from build123d import *

# Parameters (mm, degrees)
F1_DEPTH = 60
F2_R     = 11.5
F3_DEPTH = 2.5
F5_T     = -2.5
F4_R     = 1
F6_DEPTH = 25
F7_SIZE  = 1.5
F8_R     = 3.5
F8_R_2   = 5
F8_R_3   = 10
F9_DEPTH = 3


with BuildPart() as f1:
    # F0 (on Right) → F1 (new body)
    with BuildSketch(Plane.YZ):
        Polygon((30, 63), (-30, 63), (-30, 3), (0, 3), (30, 3), align=None)
    extrude(amount=F1_DEPTH)

    # F2 (on face) → F3 (cut)
    with BuildSketch(Plane(origin=(0, 0, 0), x_dir=(0, -1, 0), z_dir=(-1, 0, 0))):
        with Locations((0, 40)):
            Circle(F2_R)
    extrude(amount=-F3_DEPTH, mode=Mode.SUBTRACT)

    # F5
    f5_openings = [f1.faces().sort_by_distance(p)[0] for p in [
        (60, 0, 33),
    ]]
    offset(amount=F5_T, openings=f5_openings, kind=Kind.INTERSECTION)

    # F4 (on face) → F6 (cut)
    with BuildSketch(Plane(origin=(0, 0, 0), x_dir=(0, -1, 0), z_dir=(-1, 0, 0))):
        with Locations((0, 49.5)):
            Circle(F4_R)
        with Locations((-8.227241336, 44.75)):
            Circle(F4_R)
        with Locations((-8.227241336, 35.25)):
            Circle(F4_R)
        with Locations((0, 30.5)):
            Circle(F4_R)
        with Locations((8.227241336, 35.25)):
            Circle(F4_R)
        with Locations((8.227241336, 44.75)):
            Circle(F4_R)
    extrude(amount=-F6_DEPTH, mode=Mode.SUBTRACT)

    # F7
    f7_edges = [f1.edges().sort_by_distance(p)[0] for p in [
        (30, -30, 63),
        (30, 30, 63),
        (30, 30, 3),
        (30, -30, 3),
        (0, -30, 33),
        (0, 0, 63),
        (0, 30, 33),
        (0, 0, 3),
    ]]
    chamfer(f7_edges, length=F7_SIZE)

    # F8 (on face) → F9 (cut)
    with BuildSketch(Plane(origin=(0, 30, 0), x_dir=(-1, 0, 0), z_dir=(0, 1, 0))):
        with Locations((-50.75, 22)):
            Circle(F8_R)
        with Locations((-50.75, 33)):
            Circle(F8_R_2)
        with Locations((-30.75, 33)):
            Circle(F8_R_3)
    extrude(amount=-F9_DEPTH, mode=Mode.SUBTRACT)


solid = f1.part
Build history of the part. All positions in model axes, mm. A direction names the side the tool comes from. Coordinates: 2 decimals unless noted, no trailing zeros. Order: outer loops, then holes, each group sorted by start corner. A loop starts at its lowest first (then second) coordinate and runs counter-clockwise, first axis right, second up. Notation, with made-up numbers: (8, 35.5) - (22, 35.5) arc R24 ccw to (22, 45.5) - close; hole circle Ø2 at (-35, 45.5). An arc over 180 degrees is marked (long way). Write each question's results on one line, items separated by ' | '. Start each with the question number.
Item 1: Band-saw the part on A-A on x = 50.75. Write the cut outline in (y, z).
Item 2: Band-saw the part on C-C on x = 30.75. Write the cut outline in (y, z).
Item 3: Band-saw the part on B-B on z = 44.75. Write the cut outline in (x, y), and give its area (3 significant figures).
Item 4: Flat gauge pins, fed straight in: pin 1 (14 mm diameter, centred on y = 5.5, z = 41.5, fed in from +X); pin 2 (8 mm diameter, centred on y = -0.5, z = 14, fed in from +X); pin 3 (18.5 mm diameter, centred on y = 0, z = 40.5, fed in from -X). Where does each tip first touch, or does it go through?
Item 5: Tool access for faces 4 (the face through (2.5, 0, 40)), 5 (the face through (0, 0, 27)), 6 (the face through (30, -30, 33)), 7 (the face through (55.745, 28.768, 33.22)), 8 (the face through (2.5, -6, 27)): list every direction of +Z, -Z, +X, -X, +Y, -Y with a clear straight run to the whole face (end or side of a thin tool).
Item 6: Mould opens along Z. For faces 1 (the face through (30, 0, 3)), 2 (the face through (60, -2, 4)), 3 (the face through (31, 0, 5.5)) say: released by +Z, released by -Z, zero draft, split by the parting line, or undercut.
Item 7: Wall check: probe 1 along Z at (x, y) = (3.25, 0); probe 2 along Z at (x, y) = (50.5, -1.5); probe 3 along Y at (x, z) = (8.5, 7.5). Give the ranges that are in metal, low to high. Write a range as [from, to].
Item 8: Band-saw the part on D-D on y = 25.5. Write the cut outline in (x, z), and give its area (3 significant figures).
Numbers:
1) outline: (-30, 4.5) - (-28.5, 3) - (28.5, 3) - (30, 4.5) - (30, 18.5) - (27.5, 18.5) - (27.5, 5.5) - (-27.5, 5.5) - (-27.5, 60.5) - (27.5, 60.5) - (27.5, 38) - (30, 38) - (30, 61.5) - (28.5, 63) - (-28.5, 63) - (-30, 61.5) - close; (27.5, 25.5) - (30, 25.5) - (30, 28) - (27.5, 28) - close
2) outline: (-30, 4.5) - (-28.5, 3) - (28.5, 3) - (30, 4.5) - (30, 23) - (27.5, 23) - (27.5, 5.5) - (-27.5, 5.5) - (-27.5, 60.5) - (27.5, 60.5) - (27.5, 43) - (30, 43) - (30, 61.5) - (28.5, 63) - (-28.5, 63) - (-30, 61.5) - close
3) outline: (0, -28.5) - (1.5, -30) - (60, -30) - (60, -27.5) - (2.5, -27.5) - (2.5, -13.17) - (5, -13.17) - (5, -9.23) - (2.5, -9.23) - (2.5, -10.47) - (0, -10.47) - close; (0, 10.47) - (2.5, 10.47) - (2.5, 9.23) - (5, 9.23) - (5, 13.17) - (2.5, 13.17) - (2.5, 27.5) - (60, 27.5) - (60, 30) - (1.5, 30) - (0, 28.5) - close; (2.5, -7.23) - (5, -7.23) - (5, 7.23) - (2.5, 7.23) - close | area: 439 mm^2
4) pin 1: x = 5 | pin 2: x = 2.5 | pin 3: x = 2.5
5) face 4: -X | face 5: +Z, -Z, -X, +Y, -Y | face 6: +Z, -Z, +X, -X, -Y | face 7: +Y | face 8: +X
6) face 1: released by -Z | face 2: zero draft | face 3: undercut
7) probe 1: [3, 5.5], [26, 29.5], [31.5, 48.5], [50.5, 54], [60.5, 63] | probe 2: [3, 5.5], [60.5, 63] | probe 3: [-30, -27.5], [27.5, 30]
8) outline: (0, 4.5) - (1.5, 3) - (60, 3) - (60, 5.5) - (2.5, 5.5) - (2.5, 60.5) - (60, 60.5) - (60, 63) - (1.5, 63) - (0, 61.5) - close | area: 435 mm^2
